The listing builds one solid part. Answer for the finished solid, in the listing's coordinates (mm). Round coordinates to 2 decimals unless told otherwise and drop trailing zeros. Write each loop counter-clockwise with the first axis right and the second up, starting at its lowest first coordinate (ties: lowest second). Pieces come first, ordered by that corner, then holes. Notation, with made-up numbers: (53.25, 9.5) - (58.25, 9.5) arc R12 cw to (58.25, 15.5) - close; hole circle Ø5 at (71, -22). An arc over 180 degrees is marked (long way). Use a Markdown table: item, result. Add a question column.
1) Each of these flat-tipped pins is pushed along its axis until it touches: P1, Ø10, axis at y = -40.5, z = 35, coming from the +X side; P2, Ø10, axis at y = 42.5, z = 53, coming from the -X side; P3, Ø6, axis at y = 43, z = 123, coming from the -X side. Where does it stop, or does it pass through?
2) A cutting plane is placed at D-D (y = 50). Give the vertices of the cut face in (x, z).
3) Find the intervals of material crossed by probe 1 along Z at (x, y) = (-15, 60.5); probe 2 along Y at (x, z) = (-0.5, 94); probe 3 along X at (y, z) = (0, 91), in increasing order. Write a range as from..to.
4) Determine the mould class of faces 1 (the flat face through (-55, 5, 140)), 2 (the cylindrical face through (-24.756, -58.117, 125.481)), 3 (the flat face through (10, -59, 71)) for opening direction Z: +Z half, -Z half, draft (parallel to the pull), parting line (faces both ways), or undercut.
5) A cutting plane is placed at C-C (z = 107.5). Give the vertices of the cut face in (x, y), then the cut area to 3 significant figures.
6) A cutting plane is placed at B-B (x = -19). Give the vertices of the cut face in (y, z), then the cut area to 3 significant figures.
7) A cutting plane is placed at A-A (x = 0). Give the vertices of the cut face in (y, z), then the cut area to 3 significant figures.
```python
from build123d import *

# Parameters (mm, degrees)
ESQUISSE2_R                  = 65
ESQUISSE1_R                  = 65
ESQUISSE4_W                  = 168.541891076
ESQUISSE4_H                  = 143.597897644
ENL_V_MAT_EXTRU_2_DEPTH      = 56.0000001
COQUE2_T                     = -10
ESQUISSE5_R                  = 55
ENL_V_MAT_EXTRU_3_DEPTH      = 141
ESQUISSE6_R                  = 12.294398433
ENL_V_MAT_EXTRU_4_DEPTH      = 66
ENL_V_MAT_EXTRU_4_DEPTH_BACK = 66


with BuildPart() as part:
    # Esquisse2 → Lissage2 section 0
    with BuildSketch(Plane(origin=(0, 0, 140), x_dir=(-1, 0, 0), z_dir=(0, 0, -1))):
        Circle(ESQUISSE2_R)
    # Esquisse1 → Lissage2 section 1
    with BuildSketch(Plane.XY):
        Circle(ESQUISSE1_R)
    loft()

    # Esquisse4 → Enlèv. mat.-Extru.2 (cut, through all)
    with BuildSketch(Plane(origin=(10, 0, 0), x_dir=(0, 0, -1), z_dir=(1, 0, 0))):
        with Locations((-79.475842773, 1.247725941)):
            Rectangle(ESQUISSE4_W, ESQUISSE4_H)
    extrude(amount=ENL_V_MAT_EXTRU_2_DEPTH, mode=Mode.SUBTRACT)

    # Coque2
    coque2_openings = [part.faces().sort_by_distance(p)[0] for p in [
        (10, 7.25e-07, 70),
    ]]
    offset(amount=COQUE2_T, openings=coque2_openings)

    # Esquisse5 → Enlèv. mat.-Extru.3 (cut, through all)
    with BuildSketch(Plane.XY):
        Circle(ESQUISSE5_R)
    extrude(amount=ENL_V_MAT_EXTRU_3_DEPTH, mode=Mode.SUBTRACT)

    # Esquisse6 → Enlèv. mat.-Extru.4 (cut, two sides)
    with BuildSketch(Plane(origin=(0, 0, 0), x_dir=(1, 0, 0), z_dir=(0, 1, 0))) as enl_v_mat_extru_4_sk:
        with Locations((-15, -22)):
            Circle(ESQUISSE6_R)
        with Locations((-15, -118)):
            Circle(ESQUISSE6_R)
    extrude(amount=ENL_V_MAT_EXTRU_4_DEPTH, mode=Mode.SUBTRACT)
    extrude(enl_v_mat_extru_4_sk.sketch, amount=-ENL_V_MAT_EXTRU_4_DEPTH_BACK, mode=Mode.SUBTRACT)


solid = part.part
```
Entries:
| question | item | result |
|---|---|---|
| 1 | P1 | stops at x = -30.9 |
| 1 | P2 | stops at x = -53.09 |
| 1 | P3 | stops at x = -51.23 |
| 2 | outline | (-41.53, 0) - (-22.91, 0) - (-22.91, 12.59) arc R12.29 cw to (-22.91, 31.41) - (-22.91, 108.59) arc R12.29 cw to (-22.91, 127.41) - (-22.91, 140) - (-41.53, 140) - close |
| 3 | probe 1 | z = 0..9.71, 34.29..105.71, 130.29..140 |
| 3 | probe 2 | y = -65..-55, 55..65 |
| 3 | probe 3 | x = -65..-55 |
| 4 | face 1 | +Z half |
| 4 | face 2 | undercut |
| 4 | face 3 | draft |
| 5 | outline | (-21.4, -61.38) - (-21.4, -50.67) arc R55 cw to (-21.4, 50.67) - (-21.4, 61.38) arc R65 ccw to start; (-8.6, -64.43) arc R65 ccw to (10, -64.23) - (10, -54.08) arc R55 cw to (-8.6, -54.32) - close; (-8.6, 54.32) arc R55 cw to (10, 54.08) - (10, 64.23) arc R65 ccw to (-8.6, 64.43) - close |
| 5 | area | 1,820 mm² |
| 6 | outline | (-62.16, 0) - (-51.61, 0) - (-51.61, 10.37) - (-62.16, 10.37) - close; (-62.16, 33.63) - (-51.61, 33.63) - (-51.61, 106.37) - (-62.16, 106.37) - close; (-62.16, 129.63) - (-51.61, 129.63) - (-51.61, 140) - (-62.16, 140) - close; (51.61, 0) - (62.16, 0) - (62.16, 10.37) - (51.61, 10.37) - close; (51.61, 33.63) - (62.16, 33.63) - (62.16, 106.37) - (51.61, 106.37) - close; (51.61, 129.63) - (62.16, 129.63) - (62.16, 140) - (51.61, 140) - close |
| 6 | area | 1,970 mm² |
| 7 | outline | (-65, 0) - (-55, 0) - (-55, 140) - (-65, 140) - close; (55, 0) - (65, 0) - (65, 140) - (55, 140) - close |
| 7 | area | 2,800 mm² |
